from build123d import *

# Parameters (mm, degrees)
EXTRUDE_1_DEPTH      = 2
EXTRUDE_1_DEPTH_BACK = 20
SKETCH_1_W           = 308
SKETCH_1_H           = 78
SKETCH_1_W_2         = 300
SKETCH_1_H_2         = 70
CHAMFER_1_SIZE       = 1


with BuildPart() as part:
    # Эскиз1 → Бобышка-Вытянуть1 (new, two sides: drawn at the far end of the back side and taken through both)
    with BuildSketch(Plane.XY.offset(-EXTRUDE_1_DEPTH_BACK)):
        Rectangle(SKETCH_1_W, SKETCH_1_H)
        Rectangle(SKETCH_1_W_2, SKETCH_1_H_2, mode=Mode.SUBTRACT)
    extrude(amount=EXTRUDE_1_DEPTH + EXTRUDE_1_DEPTH_BACK)

    # Фаска1
    chamfer_1_edges = [part.edges().sort_by_distance(p)[0] for p in [
        (-150, 0, 2),
        (0, -35, 2),
        (150, 0, 2),
        (0, 35, 2),
    ]]
    chamfer(chamfer_1_edges, length=CHAMFER_1_SIZE)


solid = part.part
Source: CAD feature listing. Evaluate the final solid. Frame: model axes, mm. A direction names the side the tool comes from. Give positions to 0.01 mm unless a question says otherwise; leave off trailing zeros. Write each loop counter-clockwise with the first axis right and the second up, starting at its lowest first coordinate (ties: lowest second). Pieces come first, ordered by that corner, then holes. Notation, with made-up numbers: M 17,28 L 52,28 A28 cw 52,50 Z; hole C 57.25,-27 d10. An arc over 180 degrees is marked long. Return JSON: item names as keys, results as strings. Group by question number.
1) Cut plane B-B, the plane x = 133.5. Output: boundary loops of the cut face in (y, z), plus the area to 3 significant figures.
2) Cut plane C-C, the plane z = -16.5. Output: boundary loops of the cut face in (x, y), plus the area to 3 significant figures.
3) Set-up query: faces 1 (the face through (-2, -35, -10)), 2 (the face through (-1, 38, -20)). Return all of +Z, -Z, +X, -X, +Y, -Y with unobstructed straight access to the full face (end or side cutting, diameter ignored); none if empty.
4) Pull-direction query (Y, two-part tool) for faces 3 (the face through (150, 0, -10)), 4 (the face through (-2, 39, -9)), 5 (the face through (-1, 38, 2)); classes: pulls with the +Y half, pulls with the -Y half, needs draft (parallel to the pull), parting line crosses it, or undercut.
5) Cut plane A-A, the plane y = 19. Output: boundary loops of the cut face in (x, z), plus the area to 3 significant figures.
6) Material intervals for line 1 along Y through (x, z) = (113.5, -5.25); line 2 along X through (y, z) = (-2, 0.75), sorted ascending. Write a range as [from, to].
Recorded:
{
 "1": {"outline": "M -39,-20 L -35,-20 L -35,1 L -36,2 L -39,2 Z; M 35,-20 L 39,-20 L 39,2 L 36,2 L 35,1 Z", "area": "175 mm²"},
 "2": {"outline": "M -154,-39 L 154,-39 L 154,39 L -154,39 Z; hole M -150,-35 L 150,-35 L 150,35 L -150,35 Z", "area": "3,020 mm²"},
 "3": {"face 1": "+Z, -Z", "face 2": "-Z, +X, -X, +Y, -Y"},
 "4": {"face 3": "undercut", "face 4": "pulls with the +Y half", "face 5": "needs draft"},
 "5": {"outline": "M -154,-20 L -150,-20 L -150,1 L -151,2 L -154,2 Z; M 150,-20 L 154,-20 L 154,2 L 151,2 L 150,1 Z", "area": "175 mm²"},
 "6": {"line 1": "y = [-39, -35], [35, 39]", "line 2": "x = [-154, -150], [150, 154]"}
}
